Geometry: final body of the model. Coordinates: model frame, mm. Face numbers are marked on the shaded views. A direction names the side the tool comes from. Coordinates: 2 decimals unless noted, no trailing zeros. Order: outer loops, then holes, each group sorted by start corner. A loop starts at its lowest first (then second) coordinate and runs counter-clockwise, first axis right, second up. Notation, with made-up numbers: M 3,42 L 17,42 A32 ccw 17,77 Z; hole C 88,29.5 d10. An arc over 180 degrees is marked long. One line per question, with ' | ' between items.
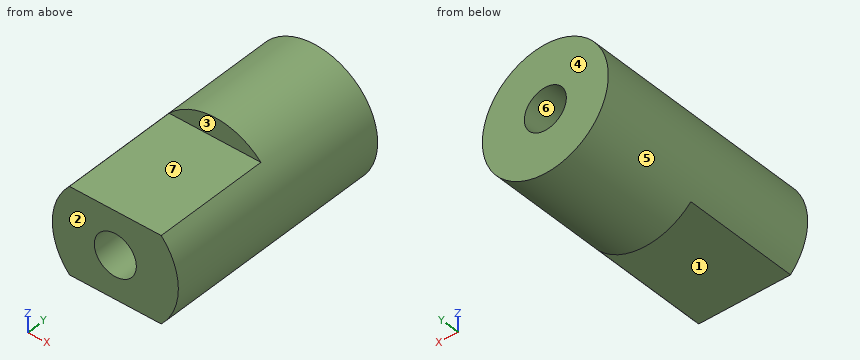
from build123d import *

# Parameters (mm, degrees)
SKETCH_R        = 2.7
PAD_DEPTH       = 10
POCKET_DEPTH    = 5
SKETCH002_R     = 0.9
POCKET001_DEPTH = 10.001


with BuildPart() as part:
    # Sketch → Pad (new body)
    with BuildSketch(Plane.XZ):
        Circle(SKETCH_R)
    extrude(amount=PAD_DEPTH)

    # Sketch001 (on Face3 of Pad) → Pocket (cut)
    with BuildSketch(Plane.XZ.offset(10)):
        with BuildLine():
            Line((-1.966596, 1.85), (1.966596, 1.85))
            ThreePointArc((1.966596, 1.85), (0, 2.7), (-1.966596, 1.85))
        make_face()
        with BuildLine():
            Line((-1.966596, -1.85), (1.966596, -1.85))
            ThreePointArc((-1.966596, -1.85), (0, -2.7), (1.966596, -1.85))
        make_face()
    extrude(amount=-POCKET_DEPTH, mode=Mode.SUBTRACT)

    # Sketch002 (on Face3 of Pocket) → Pocket001 (cut, through all)
    with BuildSketch(Plane.XZ.offset(10)):
        Circle(SKETCH002_R)
    extrude(amount=-POCKET001_DEPTH, mode=Mode.SUBTRACT)


solid = part.part
1. Pin query (flat end, axial travel): P1, Ø2, axis at y = -8.5, z = -0.5, coming from the +X side; P2, Ø3, axis at x = -0.5, y = -7.5, coming from the +Z side; P3, Ø3, axis at x = 2, y = -1.5, coming from the -Z side; P4, Ø1.2, axis at x = 0.5, y = -8.5, coming from the -Z side. Return the tip coordinate at first contact, or that it passes through.
Response values:
P1: stops at x = 2.7 | P2: stops at z = 1.85 | P3: stops at z = -2.65 | P4: stops at z = -1.85
2. Access query for the marked faces 1, 2 and 3. Directions: +Z, -Z, +X, -X, +Y, -Y. A direction counts if a zero-diameter tool reaches every point of the face in a straight line with its end or side. Return the directions, or none.
Response values:
face 1: -Z, +X, -X, -Y | face 2: +Z, -Z, +X, -X, -Y | face 3: +Z, +X, -X, -Y
3. Section B-B, the plane x = 0. Output: boundary loops of the cut face in (y, z).
Response values:
outline: M -10,-1.85 L -5,-1.85 L -5,-2.7 L 0,-2.7 L 0,-0.9 L -10,-0.9 Z; M -10,0.9 L 0,0.9 L 0,2.7 L -5,2.7 L -5,1.85 L -10,1.85 Z
4. Section C-C, the plane y = -7.75. Output: boundary loops of the cut face in (x, z).
Response values:
outline: M -1.97,-1.85 L 1.97,-1.85 A2.7 ccw 1.97,1.85 L -1.97,1.85 A2.7 ccw Z; hole C 0,0 d1.8
5. Material intervals for line 1 (Z direction, x = 0, y = -6.5); line 2 (Z direction, x = 0, y = -4); line 3 (Z direction, x = 1.75, y = -9), sorted ascending. Write a range as [from, to].
Response values:
line 1: z = [-1.85, -0.9], [0.9, 1.85] | line 2: z = [-2.7, -0.9], [0.9, 2.7] | line 3: z = [-1.85, 1.85]
6. Section A-A, the plane z = 0. Output: boundary loops of the cut face in (x, y).
Response values:
outline: M -2.7,-10 L -0.9,-10 L -0.9,0 L -2.7,0 Z; M 0.9,-10 L 2.7,-10 L 2.7,0 L 0.9,0 Z
7. Draft query along Z for the marked faces 4, 5, 6 and 7. Return one class per face: pulls with the +Z half, pulls with the -Z half, needs draft (parallel to the pull), parting line crosses it, or undercut.
Response values:
face 4: needs draft | face 5: parting line crosses it | face 6: undercut | face 7: pulls with the +Z half
8. Section D-D, the plane x = 1.7. Output: boundary loops of the cut face in (y, z).
Response values:
outline: M -10,-1.85 L -5,-1.85 L -5,-2.1 L 0,-2.1 L 0,2.1 L -5,2.1 L -5,1.85 L -10,1.85 Z
